from build123d import *

# Parameters (mm, degrees)
SKETCH1_W           = 25.4
SKETCH1_H           = 15.24
BOSS_EXTRUDE1_DEPTH = 2.794
SKETCH2_W           = 12.7
SKETCH2_H           = 15.24
BOSS_EXTRUDE2_DEPTH = 12.7
FILLET1_R           = 6.35
SKETCH3_R           = 3.175
CUT_EXTRUDE1_DEPTH  = 34.428754628
SKETCH4_R           = 1.787540604
CUT_EXTRUDE2_DEPTH  = 33.228986953


with BuildPart() as part:
    # Sketch1 → Boss-Extrude1 (new body)
    with BuildSketch(Plane(origin=(0, 0, 0), x_dir=(1, 0, 0), z_dir=(0, 1, 0))):
        with Locations((12.7, 7.62)):
            Rectangle(SKETCH1_W, SKETCH1_H)
    extrude(amount=BOSS_EXTRUDE1_DEPTH)

    # Sketch2 → Boss-Extrude2 (add)
    with BuildSketch(Plane(origin=(0, 2.794, 0), x_dir=(1, 0, 0), z_dir=(0, 1, 0))):
        with Locations((12.7, 7.62)):
            Rectangle(SKETCH2_W, SKETCH2_H)
    extrude(amount=BOSS_EXTRUDE2_DEPTH)

    # Fillet1
    fillet1_edges = [part.edges().sort_by_distance(p)[0] for p in [
        (6.35, 15.494, -7.62),
        (19.05, 15.494, -7.62),
    ]]
    fillet(fillet1_edges, radius=FILLET1_R - 0.0001)  # a hair under: the kernel refuses the full size

    # Sketch3 → Cut-Extrude1 (cut, through all)
    with BuildSketch(Plane.XY):
        with Locations((12.7, 9.144)):
            Circle(SKETCH3_R)
    extrude(amount=-CUT_EXTRUDE1_DEPTH, mode=Mode.SUBTRACT)

    # Sketch4 → Cut-Extrude2 (cut, through all)
    with BuildSketch(Plane(origin=(0, 2.794, 0), x_dir=(1, 0, 0), z_dir=(0, 1, 0))):
        with Locations(Location((3.048, 7.62, 0), (0, 0, 270))):
            Circle(SKETCH4_R)
        with Locations(Location((22.352, 7.62, 0), (0, 0, 270))):
            Circle(SKETCH4_R)
    extrude(amount=-CUT_EXTRUDE2_DEPTH, mode=Mode.SUBTRACT)


solid = part.part
Here's how the part is built. I have some questions about the finished solid (model axes, mm). A direction names the side the tool comes from. Round coordinates to 2 decimals unless told otherwise and drop trailing zeros. Order: outer loops, then holes, each group sorted by start corner. A loop starts at its lowest first (then second) coordinate and runs counter-clockwise, first axis right, second up. Notation, with made-up numbers: M 19.25,25.25 L 30.25,25.25 A14 ccw 30.25,36.25 Z; hole C -22,-18 d2. An arc over 180 degrees is marked long. Return JSON: item names as keys, results as strings. Group by question number.
1. If we section it at C-C on y = 10: List the corners of the cut face in (x, z) for me.
2. Please list where these lines run through material, in increasing order: probe 1 along X at (y, z) = (1.75, -7.62); probe 2 along Y at (x, z) = (12.7, -8.25); probe 3 along X at (y, z) = (9, -9.75).
3. I'm going to push flat-ended pins straight in: pin 1 Ø6 at (x, z) = (2.5, -3) entering from +Y; pin 2 Ø5 at (y, z) = (7, -11) entering from +X; pin 3 Ø1.5 at (x, z) = (15, -7.5) entering from -Y; pin 4 Ø3 at (x, z) = (17.5, -8.5) entering from +Y. Where does each tip first touch, or does it pass through?
4. On a 3-axis mill with a long thin cutter (end or side, diameter ignored), from which of +Z, -Z, +X, -X, +Y, -Y can I reach the whole of each face in a straight line? I mean faces 1 (the face through (3.84, 2.794, -9.42)), 2 (the face through (21.5, 2.794, -9.4)), 3 (the face through (20.607, 1.417, -8.008)). Say none if no direction works.
5. If we section it at A-A on z = -7.62: State how many separate pieces and enclosed holes the cut face has, then the cut area to 3 significant figures.
6. If we section it at B-B on x = 15.25: List the corners of the cut face in (y, z) for me, then the cut area to 3 significant figures.
7. If we mould it in two halves opening along X, with no side actions, what happens to faces 4 (the face through (13, 4, -15.24)), 5 (the face through (6.35, 6, -8)), 6 (the face through (3.127, 1.417, -9.406))? For each: pulls with the +X half, pulls with the -X half, needs draft (parallel to the pull), parting line crosses it, or undercut.
Reply:
{
 "1": {"outline": "M 6.41,-15.24 L 9.64,-15.24 L 9.64,0 L 6.41,0 Z; M 15.76,-15.24 L 18.99,-15.24 L 18.99,0 L 15.76,0 Z"},
 "2": {"probe 1": "0 to 1.26, 4.84 to 20.56, 24.14 to 25.4", "probe 2": "0 to 5.97, 12.32 to 15.49", "probe 3": "6.35 to 9.53, 15.87 to 19.05"},
 "3": {"pin 1": "y = 2.79", "pin 2": "x = 19.05", "pin 3": "y = 0", "pin 4": "y = 14.57"},
 "4": {"face 1": "+Z, -Z, -X, +Y", "face 2": "+Z, -Z, +X, +Y", "face 3": "+Y, -Y"},
 "5": {"separate pieces": "3", "enclosed holes": "1", "area": "163 mm^2"},
 "6": {"outline": "M 0,-15.24 L 7.25,-15.24 L 7.25,0 L 0,0 Z; M 11.04,-15.24 L 14.96,-15.24 L 14.96,0 L 11.04,0 Z", "area": "170 mm^2"},
 "7": {"face 4": "needs draft", "face 5": "pulls with the -X half", "face 6": "undercut"}
}
